Build history of the part. All positions in model axes, mm. Face numbers are marked on the shaded views. Coordinates: 2 decimals unless noted, no trailing zeros. Write each loop counter-clockwise with the first axis right and the second up, starting at its lowest first coordinate (ties: lowest second). Pieces come first, ordered by that corner, then holes.
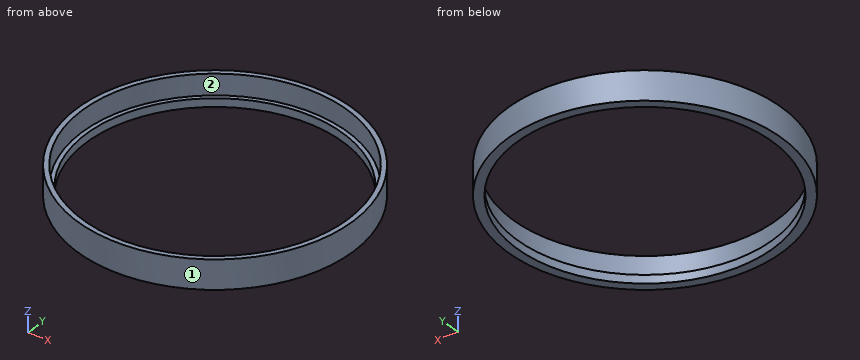
```python
from build123d import *

# Parameters (mm, degrees)
CYLINDER_R        = 77
CYLINDER_DEPTH    = 5
CYLINDER001_R     = 79.5
CYLINDER001_DEPTH = 12.5
CYLINDER002_R     = 82.5
CYLINDER002_DEPTH = 17.5


with BuildPart() as cylinder:
    # Cylinder → Cylinder (new body)
    with BuildSketch(Plane.XY):
        Circle(CYLINDER_R)
    extrude(amount=CYLINDER_DEPTH)


with BuildPart() as fusion:
    # Cylinder001 → Cylinder001 (new body)
    with BuildSketch(Plane.XY.offset(5)):
        Circle(CYLINDER001_R)
    extrude(amount=CYLINDER001_DEPTH)

    # Fusion: union Cylinder
    add(cylinder.part)


with BuildPart() as obj1:
    # Cylinder002 → Cylinder002 (new body)
    with BuildSketch(Plane.XY):
        Circle(CYLINDER002_R)
    extrude(amount=CYLINDER002_DEPTH)

    # Cut: cut Fusion
    add(fusion.part, mode=Mode.SUBTRACT)


solid = obj1.part
```
1. Saw through at C-C on z = 13.5. List the corners of the cut face in (x, y), plus the area to 3 significant figures.
Computed values:
outline: circle Ø165 at (0, 0); hole circle Ø159 at (0, 0)
area: 1,530 mm2
2. Saw through at A-A on y = 0. List the corners of the cut face in (x, z), plus the area to 3 significant figures.
Computed values:
outline: (-82.5, 0) - (-77, 0) - (-77, 5) - (-79.5, 5) - (-79.5, 17.5) - (-82.5, 17.5) - close; (77, 0) - (82.5, 0) - (82.5, 17.5) - (79.5, 17.5) - (79.5, 5) - (77, 5) - close
area: 130 mm2
3. Saw through at D-D on z = 2.25. List the corners of the cut face in (x, y).
Computed values:
outline: circle Ø165 at (0, 0); hole circle Ø154 at (0, 0)
4. Probe line 1 along Y through (x, z) = (0, 14); line 2 along Y through (x, z) = (0, 2.3); line 3 along X through (y, z) = (10, 14). List the from-to ranges inside material, lowest first.
Computed values:
line 1: y = -82.5 to -79.5, 79.5 to 82.5
line 2: y = -82.5 to -77, 77 to 82.5
line 3: x = -81.89 to -78.87, 78.87 to 81.89
5. Mould opens along X. For the marked faces 1 and 2 say: +X half, -X half, draft (parallel to the pull), parting line (faces both ways), or undercut.
Computed values:
face 1: parting line
face 2: undercut
6. Flat gauge pins, fed straight in: pin 1 (10 mm diameter, centred on x = 11, z = 7, fed in from -Y); pin 2 (3 mm diameter, centred on y = -18.5, z = 4, fed in from +X); pin 3 (10 mm diameter, centred on x = 17.5, z = 14.5, fed in from +Y). Where does each tip first touch, or does it go through?
Computed values:
pin 1: stops at y = -82.28
pin 2: stops at x = 80.73
pin 3: stops at y = 81.55
